```python
from build123d import *

# Parameters (mm, degrees)
BOSS_EXTRUDE1_DEPTH     = 40
SKETCH2_W               = 26
SKETCH2_H               = 6
CUT_EXTRUDE1_DEPTH      = 243.400412541
CUT_EXTRUDE1_DEPTH_BACK = 243.400412541
SKETCH4_R               = 2.5
SKETCH7_R               = 5
CUT_EXTRUDE3_DEPTH      = 62


with BuildPart() as part:
    # Sketch1 → Boss-Extrude1 (new body)
    with BuildSketch(Plane.XY):
        with BuildLine():
            Line((0, 0), (228.6, 0))
            Line((228.6, 0), (228.6, 70))
            ThreePointArc((228.6, 70), (114.3, 23.006536612), (0, 70))
            Line((0, 70), (0, 0))
        make_face()
    extrude(amount=BOSS_EXTRUDE1_DEPTH)

    # Sketch2 → Cut-Revolve1 (revolve, cut)
    with BuildSketch(Plane(origin=(114.3, 0, 0), x_dir=(0, 0, -1), z_dir=(1, 0, 0))):
        with Locations((-20, 12.006536612)):
            Rectangle(SKETCH2_W, SKETCH2_H)
    revolve(axis=Axis((114.3, 185.506536612, 40), (0, 0, 1)), mode=Mode.SUBTRACT)

    # Sketch4 → Cut-Extrude1 (cut, two sides: drawn at the far end of the back side and taken through both)
    with BuildSketch(Plane.XZ.offset(-CUT_EXTRUDE1_DEPTH_BACK)):
        with Locations(Location((12.7, 20, 0), (0, 0, 270))):
            Circle(SKETCH4_R)
        with Locations(Location((215.9, 20, 0), (0, 0, 270))):
            Circle(SKETCH4_R)
    extrude(amount=CUT_EXTRUDE1_DEPTH + CUT_EXTRUDE1_DEPTH_BACK, mode=Mode.SUBTRACT)

    # Sketch7 → Cut-Extrude3 (cut)
    with BuildSketch(Plane(origin=(0, 70, 0), x_dir=(-1, 0, 0), z_dir=(0, -1, 0))):
        with Locations(Location((-215.9, -20, 0), (0, 0, 270))):
            Circle(SKETCH7_R)
        with Locations(Location((-12.7, -20, 0), (0, 0, 270))):
            Circle(SKETCH7_R)
    extrude(amount=CUT_EXTRUDE3_DEPTH, mode=Mode.SUBTRACT)

    # Sketch8 → Cut-Revolve4 (revolve, cut)
    with BuildSketch(Plane(origin=(114.3, 0, 0), x_dir=(0, 0, -1), z_dir=(1, 0, 0))):
        Polygon((-7, 15.006536612), (-37, 15.006536612), (-37, 19.006536612), (0, 19.006536612), (0, -48.777467523), (-40, -48.777467523), (-40, 5.006536612), (-3, 5.006536612), (-3, 9.006536612), (-7, 9.006536612), align=None)
    revolve(axis=Axis((114.3, 185.506536612, 40), (0, 0, 1)), mode=Mode.SUBTRACT)


solid = part.part
```
Read the model definition and answer for the solid it produces. Units are mm, in the model's axes. A direction names the side the tool comes from. Round coordinates to 2 decimals unless told otherwise and drop trailing zeros. Loops run counter-clockwise (first coordinate to the right, second up) from the corner with the lowest first, then second, coordinate; pieces in that order, holes last. Notation, with made-up numbers: (23.25, -26.75) -> (71.25, -26.75) arc R12 cw to (71.25, -10.75) -> close; hole circle Ø2 at (2.5, 61). An arc over 180 degrees is marked (long way). One line per item, written item: value.
1) The mould has two halves that part along Z. Classify faces 1 (the face through (228.6, 66, 24)), 2 (the face through (114, 21, 40)), 3 (the face through (115, 12, 33)), 4 (the face through (218.9, 56.5, 16)): pulls with the +Z half, pulls with the -Z half, needs draft (parallel to the pull), parting line crosses it, or undercut.
Answer list:
face 1: needs draft
face 2: pulls with the +Z half
face 3: pulls with the -Z half
face 4: undercut
2) For faces 5 (the face through (115, 8, 3)), 6 (the face through (11.2, 56.47, 24.77)), 7 (the face through (112.546, 15.016, 35.028)), determine the directions among +Z, -Z, +X, -X, +Y, -Y from which every point of the face is accessible in a straight line to the end or side of a thin tool.
Answer list:
face 5: -Z, -Y
face 6: +Y, -Y
face 7: -Z
3) A cutting plane is placed at D-D (x = 215.9). Determine the outline of the cut face in (y, z), and give its area (3 significant figures).
Answer list:
outline: (36.32, 3) -> (41.18, 3) -> (41.18, 15) -> (36.32, 15) -> close; (36.32, 25) -> (41.18, 25) -> (41.18, 33) -> (48.58, 33) -> (48.58, 37) -> (53.6, 37) -> (53.6, 25) -> (58.69, 25) -> (58.69, 40) -> (36.32, 40) -> close; (53.6, 0) -> (58.69, 0) -> (58.69, 15) -> (53.6, 15) -> close
area: 351 mm²
4) A cutting plane is placed at B-B (y = 39). Determine the outline of the cut face in (x, z), and give its area (3 significant figures).
Answer list:
outline: (8.87, 3) -> (15.87, 3) -> (15.87, 16.13) arc R5 cw to (8.87, 16.79) -> close; (8.87, 23.21) arc R5 cw to (15.87, 23.87) -> (15.87, 33) -> (27.09, 33) -> (27.09, 37) -> (35.19, 37) -> (35.19, 0) -> (44, 0) -> (44, 40) -> (8.87, 40) -> close; (184.6, 0) -> (193.41, 0) -> (193.41, 37) -> (201.51, 37) -> (201.51, 33) -> (212.73, 33) -> (212.73, 23.87) arc R5 cw to (219.73, 23.21) -> (219.73, 40) -> (184.6, 40) -> close; (212.73, 3) -> (219.73, 3) -> (219.73, 16.79) arc R5 cw to (212.73, 16.13) -> close
area: 1,300 mm²
5) A cutting plane is placed at A-A (z = 28.5). Determine the outline of the cut face in (x, y), and give its area (3 significant figures).
Answer list:
outline: (0, 45.81) arc R180.5 ccw to (228.6, 45.81) -> (228.6, 51.02) arc R176.5 cw to (0, 51.02) -> close; (0, 64.44) arc R166.5 ccw to (228.6, 64.44) -> (228.6, 70) arc R162.5 cw to (0, 70) -> close
area: 2,000 mm²
6) A cutting plane is placed at C-C (z = 20). Determine the outline of the cut face in (x, y).
Answer list:
outline: (0, 45.81) arc R180.5 ccw to (7.7, 39.85) -> (7.7, 44.83) arc R176.5 cw to (0, 51.02) -> close; (0, 64.44) arc R166.5 ccw to (7.7, 57.61) -> (7.7, 62.86) arc R162.5 cw to (0, 70) -> close; (17.7, 33.03) arc R180.5 ccw to (210.9, 33.03) -> (210.9, 37.79) arc R176.5 cw to (17.7, 37.79) -> close; (17.7, 49.89) arc R166.5 ccw to (210.9, 49.89) -> (210.9, 54.84) arc R162.5 cw to (17.7, 54.84) -> close; (220.9, 39.85) arc R180.5 ccw to (228.6, 45.81) -> (228.6, 51.02) arc R176.5 cw to (220.9, 44.83) -> close; (220.9, 57.61) arc R166.5 ccw to (228.6, 64.44) -> (228.6, 70) arc R162.5 cw to (220.9, 62.86) -> close
7) Consider L1, parallel to X at y = 46, z = 6.5; L2, parallel to Y at x = 40.5, z = 29; L3, parallel to Z at x = 48, y = 23.5. Determine where each line is inside the solid, lowest interval first. Write a range as [from, to].
Answer list:
L1: x = [0, 6.18], [23.41, 30.97], [197.63, 205.19], [222.42, 228.6]
L2: y = [20.78, 25.18], [36.26, 40.73]
L3: z = [33, 40]
8) Flat-ended cylindrical pins translate along their axes: P1, Ø4, axis at y = 17, z = 19, coming from the -X side; P2, Ø11.5, axis at x = 215.9, z = 20, coming from the +Y side; P3, Ø11.5, axis at x = 12.7, z = 20, coming from the -Y side; P4, Ø24.5, axis at x = 144.5, y = 44, coming from the -Z side. Find the tip coordinate at first contact, or state that the pin passes through.
Answer list:
P1: stops at x = 44.62
P2: stops at y = 63.51
P3: stops at y = 32.56
P4: passes through
